Geometry: final body of the model. Coordinates: model frame, mm. Give positions to 0.01 mm unless a question says otherwise; leave off trailing zeros. Loops run counter-clockwise (first coordinate to the right, second up) from the corner with the lowest first, then second, coordinate; pieces in that order, holes last.
1. Section C-C, the plane z = 0.9. State how many separate pieces and enclosed holes the cut face has, then the cut area to 3 significant figures.
2. Section B-B, the plane x = 8. Output: boundary loops of the cut face in (y, z).
3. Section D-D, the plane x = 12. Output: boundary loops of the cut face in (y, z).
4. First-contact query: P1, Ø2.5, axis at x = -12.78, y = 15.57, coming from the +Z side; P2, Ø0.8, axis at y = 2, z = 0.5, coming from the -X side; P3, Ø0.8, axis at x = -10.5, z = 0.5, coming from the -Y side. Flat tips, straight axial feed; report the tip coordinate or a pass-through.
5. Section A-A, the plane x = 0. Output: boundary loops of the cut face in (y, z), then the cut area to 3 significant figures.
6. Material intervals for line 1 along X through (y, z) = (16.5, 1.4); line 2 along Y through (x, z) = (-14.5, 1.25); line 3 along Y through (x, z) = (1, 1.35), sorted ascending.
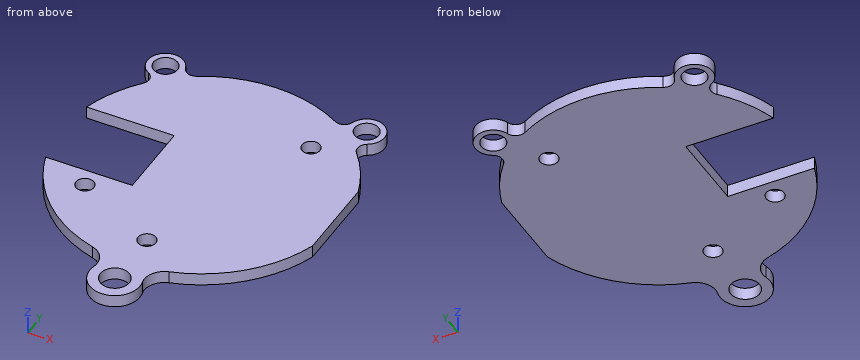
from build123d import *

# Parameters (mm, degrees)
SKETCH1_R           = 1.8415
SKETCH1_R_2         = 1.524
BOSS_EXTRUDE1_DEPTH = 1.5875
SKETCH2_R           = 1.143
CUT_EXTRUDE1_DEPTH  = 30.729408631


with BuildPart() as part:
    # Sketch1 → Boss-Extrude1 (new body)
    with BuildSketch(Plane.XY):
        with BuildLine():
            Line((-6.056265338, 4.8768), (-17.181244816, 4.8768))
            ThreePointArc((-17.181244816, 4.8768), (-15.73141865, 8.455815687), (-13.546192494, 11.63954555))
            ThreePointArc((-13.546192494, 11.63954555), (-13.259158261, 12.690113591), (-13.891550513, 13.576771304))
            ThreePointArc((-13.891550513, 13.576771304), (-14.229434947, 17.341171737), (-10.60343846, 16.274857526))
            ThreePointArc((-10.60343846, 16.274857526), (-9.857305878, 15.481530337), (-8.770915553, 15.557936625))
            ThreePointArc((-8.770915553, 15.557936625), (0, 17.859965052), (8.770915553, 15.557936625))
            ThreePointArc((8.770915553, 15.557936625), (9.857305878, 15.481530337), (10.60343846, 16.274857526))
            ThreePointArc((10.60343846, 16.274857526), (14.229434947, 17.341171737), (13.891550513, 13.576771304))
            ThreePointArc((13.891550513, 13.576771304), (13.259158261, 12.690113591), (13.546192494, 11.63954555))
            ThreePointArc((13.546192494, 11.63954555), (15.568317368, 8.752476564), (16.984058744, 5.5245))
            Line((16.984058744, 5.5245), (16.984058744, -5.5245))
            ThreePointArc((16.984058744, -5.5245), (12.377442365, -12.875452309), (4.850582957, -17.188664772))
            ThreePointArc((4.850582957, -17.188664772), (3.34119056, -18.362373067), (3.078011585, -20.256203417))
            ThreePointArc((3.078011585, -20.256203417), (0, -24.209965052), (-3.078011585, -20.256203417))
            ThreePointArc((-3.078011585, -20.256203417), (-3.34119056, -18.362373067), (-4.850582957, -17.188664772))
            ThreePointArc((-4.850582957, -17.188664772), (-12.468387001, -12.78740307), (-17.060660873, -5.2832))
            Line((-17.060660873, -5.2832), (-6.056265338, -5.2832))
            Line((-6.056265338, -5.2832), (-6.056265338, 4.8768))
        make_face()
        with Locations((0, -21.034965052)):
            Circle(SKETCH1_R, mode=Mode.SUBTRACT)
        with Locations((12.779339593, 15.573965052)):
            Circle(SKETCH1_R_2, mode=Mode.SUBTRACT)
        with Locations((-12.779339593, 15.573965052)):
            Circle(SKETCH1_R_2, mode=Mode.SUBTRACT)
    extrude(amount=BOSS_EXTRUDE1_DEPTH)

    # Sketch2 → Cut-Extrude1 (cut, through all)
    with BuildSketch(Plane.XY.offset(1.5875)):
        with Locations((8.579035657, 10.1092)):
            Circle(SKETCH2_R)
        with Locations((-10.832526773, -7.6454)):
            Circle(SKETCH2_R)
        with Locations((0, -13.2588)):
            Circle(SKETCH2_R)
    extrude(amount=-CUT_EXTRUDE1_DEPTH, mode=Mode.SUBTRACT)


solid = part.part
Answers below:
1. separate pieces: 1
1. enclosed holes: 6
1. area: 915 mm2
2. outline: (-15.97, 0) - (9.12, 0) - (9.12, 1.59) - (-15.97, 1.59) - close; (11.09, 0) - (15.97, 0) - (15.97, 1.59) - (11.09, 1.59) - close
3. outline: (-13.23, 0) - (14.26, 0) - (14.26, 1.59) - (-13.23, 1.59) - close; (16.88, 0) - (17.72, 0) - (17.72, 1.59) - (16.88, 1.59) - close
4. P1: passes through
4. P2: stops at x = -6.06
4. P3: stops at y = -14.73
5. outline: (-24.21, 0) - (-22.88, 0) - (-22.88, 1.59) - (-24.21, 1.59) - close; (-19.19, 0) - (-14.4, 0) - (-14.4, 1.59) - (-19.19, 1.59) - close; (-12.12, 0) - (17.86, 0) - (17.86, 1.59) - (-12.12, 1.59) - close
5. area: 57.3 mm2
6. line 1: x = -14.87 to -13.99, -11.57 to -10.69, -6.84 to 6.84, 10.69 to 11.57, 13.99 to 14.87
6. line 2: y = -10.43 to -5.28, 4.88 to 10.43, 14.07 to 17.08
6. line 3: y = -24.05 to -22.58, -19.49 to -13.81, -12.71 to 17.83
